Build history of the part. All positions in model axes, mm. A direction names the side the tool comes from. Give positions to 0.01 mm unless a question says otherwise; leave off trailing zeros. Loops run counter-clockwise (first coordinate to the right, second up) from the corner with the lowest first, then second, coordinate; pieces in that order, holes last. Notation, with made-up numbers: (-40, 45) -> (-12, 45) arc R36 cw to (-12, 83) -> close; hole circle Ø8 at (-32.5, 88.25). An arc over 180 degrees is marked (long way). Answer as a JSON object with one key per item and string values. Group by question number.
Q1. Drop flat-ended pins along their axis: pin 1 (4 mm diameter, centred on x = -4.5, z = 1.5, fed in from +Y); pin 2 (6 mm diameter, centred on x = 9, y = -1.5, fed in from +Z) (3 decimals); pin 3 (1 mm diameter, centred on x = 8.5, y = -2.5, fed in from -Z). Give the stop position or say it passes through.
Q2. Band-saw the part on B-B, the plane x = 7.75. Write the cut outline in (y, z) (3 decimals).
Q3. Wall check: probe 1 along X at (y, z) = (1.75, 4); probe 2 along X at (y, z) = (1.5, -2.25); probe 3 along Z at (x, y) = (4.25, 1.5). Give the ranges that are in metal, low to high. Write a range as from..to.
Q4. Band-saw the part on C-C, the plane x = -0.5. Write the cut outline in (y, z), plus the area to 3 significant figures.
Q5. Tool access for faces 1 (the flat face through (-4.73, -4.11, -2.41)), 2 (the flat face through (-4.73, 4.11, 2.41)), 3 (the flat face through (-4.731, -4.144, 2.348)), 4 (the flat face through (-4.731, 4.144, -2.348)), 5 (the cylindrical face through (6.04, -0.69, -3.1)): list every direction of +Z, -Z, +X, -X, +Y, -Y with a clear straight run to the whole face (end or side of a thin tool).
Q6. Band-saw the part on A-A, the plane x = -5.25. Write the cut outline in (y, z), plus the area to 3 significant figures.
Autodesk Inventor part; units mm, degrees
ref_plane "Work Plane1" through (10.95, 0, 0) normal (0, 0, -1) x (1, 0, 0)
ref_plane "YZ Plane" through (0, 0, 0) normal (1, 0, 0) x (0, 1, 0)
ref_plane "XZ Plane" through (0, 0, 0) normal (0, 1, 0) x (-1, 0, 0)
sketch "Sketch1" plane through (0, 0, 0) normal (0, 0, 1) x (1, 0, 0)
  line L0 (-3.2004, 0) -> (-3.2004, 3.8156)
  line L1 (0, 6.096) -> (0, 3.175)
  line L2 (1.905, 3.175) -> (12.7, 3.175)
  line L3 (12.7, 3.175) -> (12.7, 0)
  line L4 (12.7, 0) -> (-3.2004, 0)
  arc A0 (0, 6.096) -> (-1.9368, 6.5254) centre (-1.016, 6.096) ccw
  line L5 (0, -1.4605) -> (0, 8.7631)
  line L6 (-6.3805, 0) -> (15.8801, 0)
  line L7 (0, 3.175) -> (0.0001, 3.175)
  line L8 (0.0001, 3.175) -> (0.0001, 3.175)
  line L9 (0.0001, 3.175) -> (0.635, 3.175)
  line L10 (0.635, 3.175) -> (1.905, 3.175)
  line L11 (-3.2004, 3.8156) -> (-1.9368, 6.5254)
  line L12 (0.0001, 3.175) -> (1.905, 3.175) construction
  line L13 (1.905, 3.175) -> (1.905, 0) construction
  dimension "d0" = 1.016
  dimension "d1" = 12.7
  dimension "d2" = 10.795
  dimension "d3" = 14.224
  dimension "d4" = 6.35
  dimension "d5" = 3.2004
  dimension "d15" = 6.35
  dimension "d16" = 6.35
  dimension "d17" = 0.0001
  dimension "d18" = 1.27
  dimension "d19" = 25
revolve "Body" add sketch "Sketch1" angle 360 about axis through (12.7, 0, 0) along (-1, 0, 0)
sketch "Sketch2" plane through (0, 0, 0) normal (1, 0, 0) x (0, 0, -1)
  line L0 (4.7625, 2.7496) -> (4.7625, -2.7496)
  line L1 (4.7625, -2.7496) -> (0, -5.4993)
  line L2 (0, -5.4993) -> (-4.7625, -2.7496)
  line L3 (-4.7625, -2.7496) -> (-4.7625, 2.7496)
  line L4 (-4.7625, 2.7496) -> (0, 5.4993)
  line L5 (0, 5.4993) -> (4.7625, 2.7496)
  point P0 (0, 0)
  point P1 (0, 0)
  dimension "d23" = 9.525
extrude "Head" add sketch "Sketch2" against normal blind 7.112
sketch "Sketch3" plane through (0, 0, 0) normal (0, 0, 1) x (1, 0, 0)
  line L0 (-7.112, 4.7625) -> (-7.112, 5.4993)
  line L1 (-7.112, 5.4993) -> (-6.6866, 5.4993)
  line L2 (-6.6866, 5.4993) -> (-7.112, 4.7625)
  line L3 (-8.0513, 0) -> (-1.476, 0)
  line L4 (-7.112, 5.4993) -> (-7.112, 2.7496)
  line L5 (-2.4153, 5.4993) -> (-7.112, 5.4993)
  point P0 (-7.112, 2.7496)
  dimension "d8" = 30
  dimension "d22" = 9.525
revolve "Chamfer1" cut sketch "Sketch3" angle 360 about axis through (-10, 0, 0) along (1, 0, 0)
thread "Thread"
chamfer "Chamfer2" distance 0.7791 distance2 0.7791 1 edges at (12.7, -3.175, 0) measured on face at (12.7, 1.0583, 0)
ref_plane "Work Plane1" through (10.95, 0, 0) normal (0, 0, -1) x (1, 0, 0)
equation "\"d0\" = PHH"
equation "\"d1\" = NLG"
equation "\"d2\" = GEL"
equation "\"d3\" = LADI"
equation "\"d4\" = GD"
equation "\"d5\" = 0.45 * KOH"
equation "\"d15\" = SD2"
equation "\"d16\" = BDM"
equation "\"d18\" = GAL"
equation "\"d19\" = KEWI"
equation "\"d23\" = SW"
equation "\"d6\" = KOH"
equation "\"d8\" = ANG1"
equation "\"d22\" = SW0"
equation "\"d10\" = GEL"
equation "\"d13\" = -0.5 * SPD + 0.5 * GD"
equation "\"d14\" = GUL"
equation "\"NLG\" = 12.7"
equation "\"GD\" = NND"
equation "\"BDM\" = NND"
equation "\"KOH\" = 7.112"
equation "\"GEL\" = 10.795"
equation "\"LADI\" = 14.224"
equation "\"SW\" = 9.525"
equation "\"PHH\" = 1.016"
equation "\"SW0\" = SW"
equation "\"SPD\" = 4.79184"
equation "\"SD2\" = NND"
equation "\"SD\" = 0"
equation "\"ANG1\" = 30deg"
equation "\"KEWI\" = 25deg"
equation "\"GAL\" = 1.27"
equation "\"GUL\" = 0.77908"
equation "\"THREADDIA\" = 6.35"
equation "\"SDH\" = SW"
equation "\"TOA\" = 30deg"
equation "\"NND\" = 6.35"
equation "\"E0\" = 1.155 * SW"
equation "\"GD1\" = 4.79184"
properties part number "IFI 111 - 1/4-20 UNC x 0.5" material "Steel, Mild"
Worked answers:
{
 "1": {"pin 1": "y = 5.5", "pin 2": "z = 3.175", "pin 3": "z = -2.47"},
 "2": {"outline": "circle Ø6.35 at (0, 0)"},
 "3": {"probe 1": "-7.11..0", "probe 2": "-7.11..12.39", "probe 3": "-2.8..2.8"},
 "4": {"outline": "circle Ø13.94 at (0, 0)", "area": "153 mm2"},
 "5": {"face 1": "-Z, -X, -Y", "face 2": "+Z, -X, +Y", "face 3": "+Z, -X, -Y", "face 4": "-Z, -X, +Y", "face 5": "+X"},
 "6": {"outline": "(-5.5, 0) -> (-2.75, -4.76) -> (2.75, -4.76) -> (5.5, 0) -> (2.75, 4.76) -> (-2.75, 4.76) -> close", "area": "78.6 mm2"}
}
